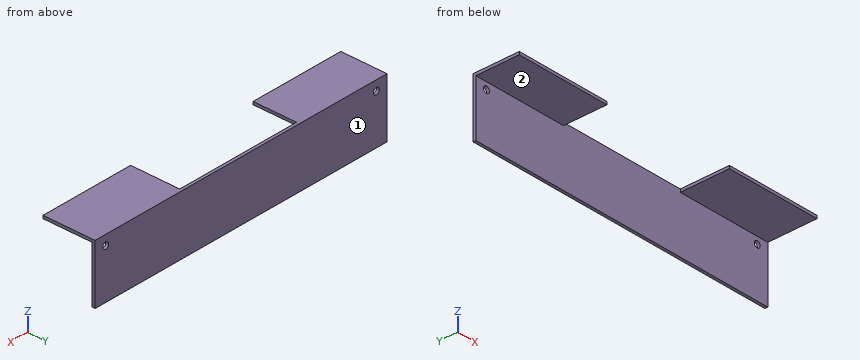
from build123d import *

# Parameters (mm, degrees)
SKETCH_1_W          = 110
SKETCH_1_H          = 19.4
EXTRUDE_1_DEPTH     = 1
SKETCH_2_W          = 33
SKETCH_2_H          = 18
EXTRUDE_2_DEPTH     = 1
SKETCH_3_W          = 33
SKETCH_3_H          = 16
EXTRUDE_3_DEPTH     = 1
SKETCH_5_W          = 44
SKETCH_5_H          = 1
EXTRUDE_5_DEPTH     = 1
SKETCH_6_R          = 1.1
CUT_EXTRUDE_1_DEPTH = 10


with BuildPart() as part:
    # 草图1 → 凸台-拉伸1 (new body)
    with BuildSketch(Plane(origin=(0, 0, 0), x_dir=(1, 0, 0), z_dir=(0, 1, 0))):
        Rectangle(SKETCH_1_W, SKETCH_1_H)
    extrude(amount=EXTRUDE_1_DEPTH)

    # 草图2 → 凸台-拉伸2 (add)
    with BuildSketch(Plane.XY.offset(9.7)):
        with Locations((38.5, -8)):
            Rectangle(SKETCH_2_W, SKETCH_2_H)
    extrude(amount=EXTRUDE_2_DEPTH)

    # 草图3 → 凸台-拉伸3 (add)
    with BuildSketch(Plane.XY.offset(9.7)):
        with Locations((-38.5, -7)):
            Rectangle(SKETCH_3_W, SKETCH_3_H)
    extrude(amount=EXTRUDE_3_DEPTH)

    # 草图5 → 凸台-拉伸5 (add)
    with BuildSketch(Plane(origin=(0, 1, 0), x_dir=(1, 0, 0), z_dir=(0, 1, 0))):
        with Locations((0, -10.2)):
            Rectangle(SKETCH_5_W, SKETCH_5_H)
    extrude(amount=-EXTRUDE_5_DEPTH)

    # 草图6 → 切除-拉伸1 (cut)
    with BuildSketch(Plane(origin=(0, 1, 0), x_dir=(1, 0, 0), z_dir=(0, 1, 0))):
        with Locations(Location((51, -7.3, 0), (0, 0, 270))):
            Circle(SKETCH_6_R)
    cut_extrude_1 = extrude(amount=-CUT_EXTRUDE_1_DEPTH, mode=Mode.SUBTRACT)

    # 镜向1: 切除-拉伸1 across plane
    add(cut_extrude_1.mirror(Plane(origin=(0, 0, 0), x_dir=(0, 0, 1), z_dir=(1, 0, 0))), mode=Mode.SUBTRACT)


solid = part.part
For this review, take the finished solid that the model builds, in its own axes (mm). Face numbers are marked on the shaded views. A direction names the side the tool comes from. Round coordinates to 2 decimals unless told otherwise and drop trailing zeros. Order: outer loops, then holes, each group sorted by start corner. A loop starts at its lowest first (then second) coordinate and runs counter-clockwise, first axis right, second up. Notation, with made-up numbers: M 4,-19 L 60,-19 A12 cw 60,-15 Z; hole C 45.25,66 d11. An arc over 180 degrees is marked long. Use a Markdown table: item, result. Add a question column.
Item 1: Add section B-B, the plane y = -12.75. Give the boundary of the cut face in (x, z).
Item 2: Tool access review of the marked faces 1 and 2: name each direction out of +Z, -Z, +X, -X, +Y, -Y from which nothing blocks a thin tool from reaching the whole face with its end or side.
Item 3: Add section A-A, the plane z = 7.3. Give the boundary of the cut face in (x, y), then the cut area to 3 significant figures.
Item 4: To check wall thickness, follow line 1 along X through (y, z) = (0.4, 7.3); line 2 along Z through (x, y) = (-45, -10); line 3 along Y through (x, z) = (-28, 4). State the ranges of each line that lie inside material, in increasing order.
Item 5: Insertion check: pin 1 (2 mm diameter, centred on y = -4, z = 8.5, fed in from -X); pin 2 (3 mm diameter, centred on x = -51, z = 7.3, fed in from -Y); pin 3 (5 mm diameter, centred on x = 36, y = -7.5, fed in from -Z); pin 4 (0.5 mm diameter, centred on x = -44, z = 10, fed in from -Y). Each pin has a flat end and moves straight along its axis. Give the tip position at first contact, or say it passes through.
Item 6: Add section C-C, the plane x = -51. Give the boundary of the cut face in (y, z), then the cut area to 3 significant figures.
Item 7: Add section D-D, the plane x = 51. Give the boundary of the cut face in (y, z), then the cut area to 3 significant figures.
Geometry results:
| question | item | result |
|---|---|---|
| 1 | outline | M -55,9.7 L -22,9.7 L -22,10.7 L -55,10.7 Z; M 22,9.7 L 55,9.7 L 55,10.7 L 22,10.7 Z |
| 2 | face 1 | +Z, -Z, +X, -X, +Y |
| 2 | face 2 | -Z, +X, -X, -Y |
| 3 | outline | M -55,0 L -52.1,0 L -52.1,1 L -55,1 Z; M -49.9,0 L 49.9,0 L 49.9,1 L -49.9,1 Z; M 52.1,0 L 55,0 L 55,1 L 52.1,1 Z |
| 3 | area | 106 mm² |
| 4 | line 1 | x = -55 to -52.1, -49.9 to 49.9, 52.1 to 55 |
| 4 | line 2 | z = 9.7 to 10.7 |
| 4 | line 3 | y = 0 to 1 |
| 5 | pin 1 | passes through |
| 5 | pin 2 | stops at y = 0 |
| 5 | pin 3 | stops at z = 9.7 |
| 5 | pin 4 | stops at y = -15 |
| 6 | outline | M -15,9.7 L 0,9.7 L 0,8.4 L 1,8.4 L 1,10.7 L -15,10.7 Z; M 0,-9.7 L 1,-9.7 L 1,6.2 L 0,6.2 Z |
| 6 | area | 33.2 mm² |
| 7 | outline | M -17,9.7 L 0,9.7 L 0,8.4 L 1,8.4 L 1,10.7 L -17,10.7 Z; M 0,-9.7 L 1,-9.7 L 1,6.2 L 0,6.2 Z |
| 7 | area | 35.2 mm² |
